from build123d import *

# Parameters (mm, degrees)
SKETCH1_W           = 10
SKETCH1_H           = 10
BOSS_EXTRUDE1_DEPTH = 310
CUT_EXTRUDE1_DEPTH  = 310
FILLET1_R           = 1
FILLET2_R           = 1
FILLET3_R           = 1
FILLET4_R           = 1
BOSS_EXTRUDE2_DEPTH = 42
CUT_EXTRUDE2_DEPTH  = 35.07
CUT_EXTRUDE3_DEPTH  = 2
BOSS_EXTRUDE4_DEPTH = 370
CUT_EXTRUDE4_DEPTH  = 46.92
SKETCH14_W          = 1
SKETCH14_H          = 46.92
CUT_EXTRUDE5_DEPTH  = 46.92


with BuildPart() as part:
    # Sketch1 → Boss-Extrude1 (new body)
    with BuildSketch(Plane(origin=(0, 0, 0), x_dir=(1, 0, 0), z_dir=(0, 1, 0))):
        with Locations((-3.5625, -0.78125)):
            Rectangle(SKETCH1_W, SKETCH1_H)
    extrude(amount=BOSS_EXTRUDE1_DEPTH)

    # Sketch2 → Cut-Extrude1 (cut)
    with BuildSketch(Plane(origin=(0, 0, 0), x_dir=(-1, 0, 0), z_dir=(0, -1, 0))):
        Polygon((-0.4375, -4.78125), (7.5625, -4.78125), (-0.4375, 3.21875), align=None)
        Polygon((-0.4375, 3.21875), (7.5625, -4.78125), (7.5625, 3.21875), align=None)
    extrude(amount=-CUT_EXTRUDE1_DEPTH, mode=Mode.SUBTRACT)

    # Fillet1
    fillet1_edges = [part.edges().sort_by_distance(p)[0] for p in [
        (0.4375, 155, -3.21875),
        (-8.5625, 155, 5.78125),
        (-8.5625, 155, -4.21875),
        (1.4375, 155, 5.78125),
    ]]
    fillet(fillet1_edges, radius=FILLET1_R)

    # Fillet2
    fillet2_edges = [part.edges().sort_by_distance(p)[0] for p in [
        (-7.5625, 155, 4.78125),
        (1.4375, 155, -4.21875),
    ]]
    fillet(fillet2_edges, radius=FILLET2_R)

    # Fillet3
    fillet3_edges = [part.edges().sort_by_distance(p)[0] for p in [
        (0.4375, 155, 4.78125),
    ]]
    fillet(fillet3_edges, radius=FILLET3_R)

    # Fillet4
    fillet4_edges = [part.edges().sort_by_distance(p)[0] for p in [
        (-7.5625, 155, -3.21875),
    ]]
    fillet(fillet4_edges, radius=FILLET4_R)

    # Sketch3 → Boss-Extrude2 (add)
    with BuildSketch(Plane(origin=(0, 310, 0), x_dir=(1, 0, 0), z_dir=(0, 1, 0))):
        with BuildLine():
            ThreePointArc((0.4375, -5.78125), (1.144606781, -5.488356781), (1.4375, -4.78125))
            Line((1.4375, -4.78125), (1.4375, 3.21875))
            ThreePointArc((1.4375, 3.21875), (1.144606781, 3.925856781), (0.4375, 4.21875))
            Line((0.4375, 4.21875), (-7.5625, 4.21875))
            ThreePointArc((-7.5625, 4.21875), (-8.269606781, 3.925856781), (-8.5625, 3.21875))
            Line((-8.5625, 3.21875), (-8.5625, -4.78125))
            ThreePointArc((-8.5625, -4.78125), (-8.269606781, -5.488356781), (-7.5625, -5.78125))
            Line((-7.5625, -5.78125), (0.4375, -5.78125))
        make_face()
        with BuildLine():
            ThreePointArc((-0.5625, 3.21875), (0.144606781, 2.925856781), (0.4375, 2.21875))
            Line((0.4375, 2.21875), (0.4375, -3.78125))
            ThreePointArc((0.4375, -3.78125), (0.144606781, -4.488356781), (-0.5625, -4.78125))
            Line((-0.5625, -4.78125), (-6.5625, -4.78125))
            ThreePointArc((-6.5625, -4.78125), (-7.269606781, -4.488356781), (-7.5625, -3.78125))
            Line((-7.5625, -3.78125), (-7.5625, 2.21875))
            ThreePointArc((-7.5625, 2.21875), (-7.269606781, 2.925856781), (-6.5625, 3.21875))
            Line((-6.5625, 3.21875), (-0.5625, 3.21875))
        make_face(mode=Mode.SUBTRACT)
    extrude(amount=BOSS_EXTRUDE2_DEPTH)

    # Sketch4 → Cut-Extrude2 (cut)
    with BuildSketch(Plane(origin=(0, 352, 0), x_dir=(1, 0, 0), z_dir=(0, 1, 0))):
        with BuildLine():
            Line((-7.5625, -5.78125), (0.4375, -5.78125))
            ThreePointArc((0.4375, -5.78125), (1.144606781, -5.488356781), (1.4375, -4.78125))
            Line((1.4375, -4.78125), (1.4375, 3.21875))
            ThreePointArc((1.4375, 3.21875), (1.144606781, 3.925856781), (0.4375, 4.21875))
            Line((0.4375, 4.21875), (-7.5625, 4.21875))
            ThreePointArc((-7.5625, 4.21875), (-8.269606781, 3.925856781), (-8.5625, 3.21875))
            Line((-8.5625, 3.21875), (-8.5625, -4.78125))
            ThreePointArc((-8.5625, -4.78125), (-8.269606781, -5.488356781), (-7.5625, -5.78125))
        make_face()
        with BuildLine():
            Line((-6.5625, 3.21875), (-0.5625, 3.21875))
            ThreePointArc((-0.5625, 3.21875), (0.144606781, 2.925856781), (0.4375, 2.21875))
            Line((0.4375, 2.21875), (0.4375, -3.78125))
            ThreePointArc((0.4375, -3.78125), (0.144606781, -4.488356781), (-0.5625, -4.78125))
            Line((-0.5625, -4.78125), (-6.5625, -4.78125))
            ThreePointArc((-6.5625, -4.78125), (-7.269606781, -4.488356781), (-7.5625, -3.78125))
            Line((-7.5625, -3.78125), (-7.5625, 2.21875))
            ThreePointArc((-7.5625, 2.21875), (-7.269606781, 2.925856781), (-6.5625, 3.21875))
        make_face(mode=Mode.SUBTRACT)
    extrude(amount=-CUT_EXTRUDE2_DEPTH, mode=Mode.SUBTRACT)

    # Sketch6 → Cut-Extrude3 (cut)
    with BuildSketch(Plane(origin=(0, 316.93, 0), x_dir=(1, 0, 0), z_dir=(0, 1, 0))):
        with BuildLine():
            Line((-7.5625, -5.78125), (0.4375, -5.78125))
            ThreePointArc((0.4375, -5.78125), (1.144606781, -5.488356781), (1.4375, -4.78125))
            Line((1.4375, -4.78125), (1.4375, 3.21875))
            ThreePointArc((1.4375, 3.21875), (1.144606781, 3.925856781), (0.4375, 4.21875))
            Line((0.4375, 4.21875), (-7.5625, 4.21875))
            ThreePointArc((-7.5625, 4.21875), (-8.269606781, 3.925856781), (-8.5625, 3.21875))
            Line((-8.5625, 3.21875), (-8.5625, -4.78125))
            ThreePointArc((-8.5625, -4.78125), (-8.269606781, -5.488356781), (-7.5625, -5.78125))
        make_face()
    extrude(amount=-CUT_EXTRUDE3_DEPTH, mode=Mode.SUBTRACT)

    # Sketch7 → Boss-Extrude4 (add)
    with BuildSketch(Plane(origin=(0, 314.93, 0), x_dir=(1, 0, 0), z_dir=(0, 1, 0))):
        with BuildLine():
            Line((-8.5625, 3.21875), (-8.5625, -4.78125))
            ThreePointArc((-8.5625, -4.78125), (-8.269606781, -5.488356781), (-7.5625, -5.78125))
            Line((-7.5625, -5.78125), (0.4375, -5.78125))
            ThreePointArc((0.4375, -5.78125), (1.144606781, -5.488356781), (1.4375, -4.78125))
            Line((1.4375, -4.78125), (1.4375, 3.21875))
            ThreePointArc((1.4375, 3.21875), (1.144606781, 3.925856781), (0.4375, 4.21875))
            Line((0.4375, 4.21875), (-7.5625, 4.21875))
            ThreePointArc((-7.5625, 4.21875), (-8.269606781, 3.925856781), (-8.5625, 3.21875))
        make_face()
        with BuildLine():
            Line((-6.5625, 3.21875), (-0.5625, 3.21875))
            ThreePointArc((-0.5625, 3.21875), (0.144606781, 2.925856781), (0.4375, 2.21875))
            Line((0.4375, 2.21875), (0.4375, -3.78125))
            ThreePointArc((0.4375, -3.78125), (0.144606781, -4.488356781), (-0.5625, -4.78125))
            Line((-0.5625, -4.78125), (-6.5625, -4.78125))
            ThreePointArc((-6.5625, -4.78125), (-7.269606781, -4.488356781), (-7.5625, -3.78125))
            Line((-7.5625, -3.78125), (-7.5625, 2.21875))
            ThreePointArc((-7.5625, 2.21875), (-7.269606781, 2.925856781), (-6.5625, 3.21875))
        make_face(mode=Mode.SUBTRACT)
    extrude(amount=-BOSS_EXTRUDE4_DEPTH)

    # Sketch13 → Cut-Extrude4 (cut)
    with BuildSketch(Plane(origin=(0, -55.07, 0), x_dir=(-1, 0, 0), z_dir=(0, -1, 0))):
        with BuildLine():
            Line((6.7625, -4.78125), (7.5625, -5.78125))
            ThreePointArc((7.5625, -5.78125), (8.269606781, -5.488356781), (8.5625, -4.78125))
            Line((8.5625, -4.78125), (8.5625, 3.21875))
            ThreePointArc((8.5625, 3.21875), (8.269606781, 3.925856781), (7.5625, 4.21875))
            Line((7.5625, 4.21875), (3.5625, 4.21875))
            Line((3.5625, 4.21875), (3.5625, 3.21875))
            Line((3.5625, 3.21875), (6.5625, 3.21875))
            Line((6.5625, 3.21875), (7.5625, 3.21875))
            Line((7.5625, 3.21875), (7.5625, 2.21875))
            Line((7.5625, 2.21875), (7.5625, -3.78125))
            Line((7.5625, -3.78125), (7.5625, -4.78125))
            Line((7.5625, -4.78125), (6.7625, -4.78125))
        make_face()
        with BuildLine():
            Line((-0.4375, -5.78125), (7.5625, -5.78125))
            Line((7.5625, -5.78125), (6.7625, -4.78125))
            Line((6.7625, -4.78125), (6.5625, -4.78125))
            Line((6.5625, -4.78125), (0.5625, -4.78125))
            Line((0.5625, -4.78125), (-0.4375, -4.78125))
            Line((-0.4375, -4.78125), (-0.4375, -3.78125))
            Line((-0.4375, -3.78125), (-0.4375, 2.21875))
            Line((-0.4375, 2.21875), (-0.4375, 3.21875))
            Line((-0.4375, 3.21875), (0.3625, 3.21875))
            Line((0.3625, 3.21875), (-0.4375, 4.21875))
            ThreePointArc((-0.4375, 4.21875), (-1.144606781, 3.925856781), (-1.4375, 3.21875))
            Line((-1.4375, 3.21875), (-1.4375, -4.78125))
            ThreePointArc((-1.4375, -4.78125), (-1.144606781, -5.488356781), (-0.4375, -5.78125))
        make_face()
        Polygon((-0.4375, 4.21875), (0.3625, 3.21875), (0.5625, 3.21875), (3.5625, 3.21875), (3.5625, 4.21875), align=None)
    extrude(amount=-CUT_EXTRUDE4_DEPTH, mode=Mode.SUBTRACT)

    # Sketch14 → Cut-Extrude5 (cut)
    with BuildSketch(Plane(origin=(0.4375, 0, 0), x_dir=(0, 0, -1), z_dir=(1, 0, 0))):
        with Locations((-4.28125, -31.61)):
            Rectangle(SKETCH14_W, SKETCH14_H)
        with Locations((2.71875, -31.61)):
            Rectangle(SKETCH14_W, SKETCH14_H)
    extrude(amount=-CUT_EXTRUDE5_DEPTH, mode=Mode.SUBTRACT)


solid = part.part
Verification items for the finished model (mm, model axes). A direction names the side the tool comes from. Coordinates: 2 decimals unless noted, no trailing zeros. Order: outer loops, then holes, each group sorted by start corner. A loop starts at its lowest first (then second) coordinate and runs counter-clockwise, first axis right, second up. Notation, with made-up numbers: M 75.5,46.25 L 101.5,46.25 A14 ccw 101.5,61.25 Z; hole C -14,-25 d2. An arc over 180 degrees is marked long. Return JSON: item names as keys, results as strings.
1) Release check for a two-part mould opening along X. For faces 3 (the flat face through (-7.562, 151, 1)), 4 (the flat face through (1.438, 151, 1)), 5 (the flat face through (-8, -8.15, 1)), 6 (the flat face through (-8.562, 151, 1)) record: +X half, -X half, draft (parallel to the pull), parting line (faces both ways), or undercut.
Answer list:
{"face 3": "undercut", "face 4": "+X half", "face 5": "draft", "face 6": "-X half"}
2) Cross-section at B-B, the plane y = 276. Record the boundary of the cut face in (x, z).
Answer list:
{"outline": "M -8.56,-3.22 A1 ccw -7.56,-4.22 L 0.44,-4.22 A1 ccw 1.44,-3.22 L 1.44,4.78 A1 ccw 0.44,5.78 L -7.56,5.78 A1 ccw -8.56,4.78 Z; hole M -7.56,-2.22 A1 ccw -6.56,-3.22 L -0.56,-3.22 A1 ccw 0.44,-2.22 L 0.44,3.78 A1 ccw -0.56,4.78 L -6.56,4.78 A1 ccw -7.56,3.78 Z"}
3) Thickness scan on L1, parallel to X at y = 32, z = -1.25; L2, parallel to Z at x = -5, y = 270; L3, parallel to X at y = 211, z = 4. Record the ranges inside material, lowest first. Write a range as [from, to].
Answer list:
{"L1": "[-8.56, -7.56], [0.44, 1.44]", "L2": "[-4.22, -3.22], [4.78, 5.78]", "L3": "[-8.56, -7.54], [0.41, 1.44]"}
4) Access from +Z, -Z, +X, -X, +Y, -Y to the whole of each face (thin tool, end or side, straight path). Record for faces 1 (the flat face through (-4, 151, 4.781)), 2 (the flat face through (-4, 151, 5.781)).
Answer list:
{"face 1": "+Y, -Y", "face 2": "+Z, +X, -X, +Y, -Y"}
5) Cross-section at A-A, the plane z = 1. Record the boundary of the cut face in (x, y), and give its area (3 significant figures).
Answer list:
{"outline": "M -8.56,-8.15 L -7.56,-8.15 L -7.56,314.93 L -8.56,314.93 Z; M 0.44,-8.15 L 1.44,-8.15 L 1.44,314.93 L 0.44,314.93 Z", "area": "646 mm2"}
